Work out the finished part from the listing and answer in its coordinate system (mm). A direction names the side the tool comes from. Round coordinates to 2 decimals unless told otherwise and drop trailing zeros. Order: outer loops, then holes, each group sorted by start corner. A loop starts at its lowest first (then second) coordinate and runs counter-clockwise, first axis right, second up. Notation, with made-up numbers: M -7,31.25 L 34,31.25 A31 ccw 34,56.25 Z; hole C -14.5,77.5 d10. An arc over 180 degrees is marked long. Return JSON: item names as keys, results as strings.
from build123d import *
from build123d.topology import SkipClean

# Parameters (mm, degrees)
SKETCH1_R                = 5.5
GEARPLATE_DEPTH          = 1.5
BOSS_EXTRUDE3_DEPTH      = 1.5
CIRPATTERN2_COUNT        = 12
SKETCH3_R                = 4.5
BACKPLATE_DEPTH          = 4
SKETCH4_R                = 5.5
PLATE_DEPTH              = 1
SKETCH6_R                = 10
ANGLEPLATE_DEPTH         = 2.5
ANGLEPLATE_DRAFT         = -35
SKETCH8_R                = 9
SMALLANGLEPLATE_DEPTH    = 0.2
SMALLANGLEPLATE_DRAFT    = 79
SKETCH9_R                = 5.5
DOMEEXTRUDE_DEPTH        = 0.5
CUT_EXTRUDE1_DEPTH       = 3.8
BOSS_EXTRUDE5_REACH      = 34.569
BOSS_EXTRUDE5_END_RADIUS = 10.833333333
SKETCH12_R               = 2.5
SKETCH15_R               = 2.5
BOSS_EXTRUDE6_DEPTH      = 5
SKETCH16_R               = 6
BOSS_EXTRUDE7_DEPTH      = 5
FILLET1_R                = 1


# Read off the part's stored shape, not the designer's step: Dome1
with BuildPart() as part:
    # Sketch1 → GearPlate (new body)
    with BuildSketch(Plane.XY):
        Circle(SKETCH1_R)
    extrude(amount=GEARPLATE_DEPTH)

    # Sketch2 → Boss-Extrude3 (add)
    with BuildSketch(Plane.XY.offset(1.5)):
        with BuildLine():
            Line((-1.157942076, 5.376724853), (1.157942076, 5.376724853))
            add(Edge.make_bspline(
                [(-1.157942076, 5.376724853), (0, 15.022701543), (1.157942076, 5.376724853)],
                knots=[0, 0, 0, 1, 1, 1], degree=2))
        make_face()
    boss_extrude3 = extrude(amount=-BOSS_EXTRUDE3_DEPTH)

    # CirPattern2: Boss-Extrude3 ×12 about axis
    cirpattern2_axis = Axis((0, 0, 1.5), (0, 0, -1))
    for i in range(1, CIRPATTERN2_COUNT):
        add(boss_extrude3.rotate(cirpattern2_axis, i * 360 / CIRPATTERN2_COUNT))

    # Sketch3 → BackPlate (add)
    with BuildSketch(Plane(origin=(0, 0, 0), x_dir=(-1, 0, 0), z_dir=(0, 0, -1))):
        with Locations(Location((0, 0, 0), (0, 0, 180))):
            Circle(SKETCH3_R)
    extrude(amount=BACKPLATE_DEPTH)

    # Sketch4 → Plate (add)
    with BuildSketch(Plane.XY.offset(1.5)):
        with Locations(Location((0, 0, 0), (0, 0, 192.153701922))):
            Circle(SKETCH4_R)
    extrude(amount=PLATE_DEPTH)


with BuildPart() as angleplate_tool:
    # Sketch6 → AnglePlate (with draft: the straight prism first)
    with BuildSketch(Plane.XY.offset(5)):
        Circle(SKETCH6_R)
    extrude(amount=-ANGLEPLATE_DEPTH)
    # AnglePlate: the draft: its side faces are tilted about the plane it starts from
    angleplate_sides = [angleplate_tool.faces().sort_by_distance(p)[0] for p in [
        (-10, 0, 3.75),
    ]]
    draft(angleplate_sides, Plane.XY.offset(5), ANGLEPLATE_DRAFT)


with BuildPart() as part_1:
    add(part.part)

    # AnglePlate: add angleplate_tool
    add(angleplate_tool.part)


with BuildPart() as smallangleplate_tool:
    # Sketch8 → SmallAnglePlate (with draft: the straight prism first)
    with BuildSketch(Plane.XY.offset(5.2)):
        Circle(SKETCH8_R)
    extrude(amount=-SMALLANGLEPLATE_DEPTH)
    # SmallAnglePlate: the draft: its side faces are tilted about the plane it starts from
    smallangleplate_sides = [smallangleplate_tool.faces().sort_by_distance(p)[0] for p in [
        (-9, 0, 5.1),
    ]]
    draft(smallangleplate_sides, Plane.XY.offset(5.2), SMALLANGLEPLATE_DRAFT)


with BuildPart() as part_2:
    add(part_1.part)

    # SmallAnglePlate: add smallangleplate_tool
    add(smallangleplate_tool.part)

    # Sketch9 → DomeExtrude (add)
    with SkipClean():  # the faces are left unmerged after this step: merging them gives an invalid solid
        with BuildSketch(Plane.XY.offset(5.2)):
            with Locations(Location((0, 0, 0), (0, 0, 192.153701922))):
                Circle(SKETCH9_R)
        extrude(amount=DOMEEXTRUDE_DEPTH)

    # Dome1 outline → Dome1 (revolve)
    with SkipClean():  # the faces are left unmerged after this step: merging them gives an invalid solid
        with BuildSketch(Plane.XZ):
            with BuildLine():
                Line((0, 5.7), (5.500000009, 5.699999994))
                ThreePointArc((5.500000009, 5.699999994), (2.850438568, 6.818274729), (0, 7.2))
                Line((0, 7.2), (0, 5.7))
            make_face()
        revolve(axis=Axis((0, 0, 0), (0, 0, 1)))

    # Sketch11 → Cut-Extrude1 (cut)
    with SkipClean():  # the faces are left unmerged after this step: merging them gives an invalid solid
        with BuildSketch(Plane.XY.offset(10.2)):
            Polygon((-0.75, 2), (0.75, 2), (0.75, 0.75), (2, 0.75), (2, -0.75), (0.75, -0.75), (0.75, -2), (-0.75, -2), (-0.75, -0.75), (-2, -0.75), (-2, 0.75), (-0.75, 0.75), align=None)
        extrude(amount=-CUT_EXTRUDE1_DEPTH, mode=Mode.SUBTRACT)

    # Boss-Extrude5: up to this sphere (the profile starts outside it)
    with SkipClean():  # the faces are left unmerged after this step: merging them gives an invalid solid
        boss_extrude5_end = Location((0, 0, -3.633333333)) * Sphere(BOSS_EXTRUDE5_END_RADIUS, mode=Mode.PRIVATE)
        # Sketch12 → Boss-Extrude5 (add, up to the surface)
        with BuildSketch(Plane.XY.offset(25.2), mode=Mode.PRIVATE) as boss_extrude5_sk1:
            Circle(SKETCH12_R)
        boss_extrude5_tool1 = extrude(boss_extrude5_sk1.sketch, amount=-BOSS_EXTRUDE5_REACH, mode=Mode.PRIVATE) - boss_extrude5_end
        add(boss_extrude5_tool1.solids().sort_by_distance((0, 0, 25.2))[0])

    # Sketch15 → Boss-Extrude6 (add)
    with SkipClean():  # the faces are left unmerged after this step: merging them gives an invalid solid
        with BuildSketch(Plane(origin=(0, 0, 0), x_dir=(1, 0, 0), z_dir=(0, 1, 0))):
            with Locations(Location((0, -22.2, 0), (0, 0, 270))):
                Circle(SKETCH15_R)
        extrude(amount=-BOSS_EXTRUDE6_DEPTH)

    # Sketch16 → Boss-Extrude7 (add)
    with SkipClean():  # the faces are left unmerged after this step: merging them gives an invalid solid
        with BuildSketch(Plane.XZ.offset(5)):
            with Locations(Location((0, 22.2, 0), (0, 0, 270))):
                Circle(SKETCH16_R)
        extrude(amount=BOSS_EXTRUDE7_DEPTH)

    # Fillet1
    fillet1_edges = [part_2.edges().sort_by_distance(p)[0] for p in [
        (0, -5, 28.2),
    ]]
    fillet(fillet1_edges, radius=FILLET1_R)


solid = part_2.part
Item 1: Find section A-A (z = 22.2). Determine the outline of the cut face in (x, y).
Output:
{"outline": "M -6,-10 L 6,-10 L 6,-6 A1 ccw 5,-5 L 2.5,-5 L 2.5,0 A2.5 ccw -2.5,0 L -2.5,-5 L -5,-5 A1 ccw -6,-6 Z"}
Item 2: Which of the six approach directions +Z, -Z, +X, -X, +Y, -Y give full straight-line access (tool end or side, diameter ignored) to faces 4 (the cylindrical face through (-5.41, 0.99, 5.45)), 5 (the flat face through (-4, -6, 1.5)), 6 (the flat face through (-4, 6, 1.5)), 7 (the flat face through (4, -6, 1.5)), 8 (the flat face through (4, 6, 1.5))?
Output:
{"face 4": "none", "face 5": "-X, -Y", "face 6": "-X, +Y", "face 7": "+X, -Y", "face 8": "+X, +Y"}
Item 3: Find section B-B (y = -7). State how many separate pieces and enclosed holes the cut face has, plus the area to 3 significant figures.
Output:
{"separate pieces": "5", "enclosed holes": "0", "area": "153 mm^2"}
Item 4: Each of these flat-tipped pins is pushed along its axis until it touches: pin 1 (0.8 mm diameter, centred on x = 1, z = 6.5, fed in from -Y); pin 2 (2 mm diameter, centred on x = -4.5, z = 19.5, fed in from -Y); pin 3 (0.7 mm diameter, centred on x = 7, y = -0.5, fed in from +Z); pin 4 (1 mm diameter, centred on x = -7.5, z = 19.5, fed in from -Y). Where does it stop, or does it pass through?
Output:
{"pin 1": "stops at y = -4.65", "pin 2": "stops at y = -10", "pin 3": "stops at z = 5.2", "pin 4": "passes through"}
Item 5: The mould has two halves that part along Z. Classify faces 1 (the cylindrical face through (-3.32, -3.04, -1.97)), 2 (the flat face through (0, 0, 25.2)), 3 (the flat face through (5.4, -1.7, 2.5)): pulls with the +Z half, pulls with the -Z half, needs draft (parallel to the pull), parting line crosses it, or undercut.
Output:
{"face 1": "needs draft", "face 2": "pulls with the +Z half", "face 3": "undercut"}
Item 6: Consider line 1 along Z through (x, y) = (5.25, -3.25); line 2 along Z through (x, y) = (-4, -6.25); line 3 along Z through (x, y) = (-4.5, -8.25). Determine where each line is inside the solid, lowest interval first. Write a range as [from, to].
Output:
{"line 1": "z = [0, 1.5], [2.5, 5.2]", "line 2": "z = [0, 1.5], [2.5, 5.2], [17.73, 26.67]", "line 3": "z = [0, 1.5], [4.14, 5.12], [18.23, 26.17]"}
Item 7: Find section D-D (z = 15). Determine the outline of the cut face in (x, y), plus the area to 3 significant figures.
Output:
{"outline": "C 0,0 d5", "area": "19.6 mm^2"}
